Geometry: see drawing. Coordinates: mm, zero at the bounding-box minimum. Give positions to 0.01 mm unless a question says otherwise; leave off trailing zeros. Write each loop counter-clockwise with the first axis right and the second up, starting at its lowest first coordinate (ties: lowest second). Pieces come first, ordered by that corner, then holes. Notation, with made-up numbers: M 52,66.25 L 95,66.25 A13 ccw 95,76.25 Z; hole C 49,86.5 d1. An arc over 180 degrees is marked long. Use CSV: the item, a comma, the result in double quotes. Start each with the question number.
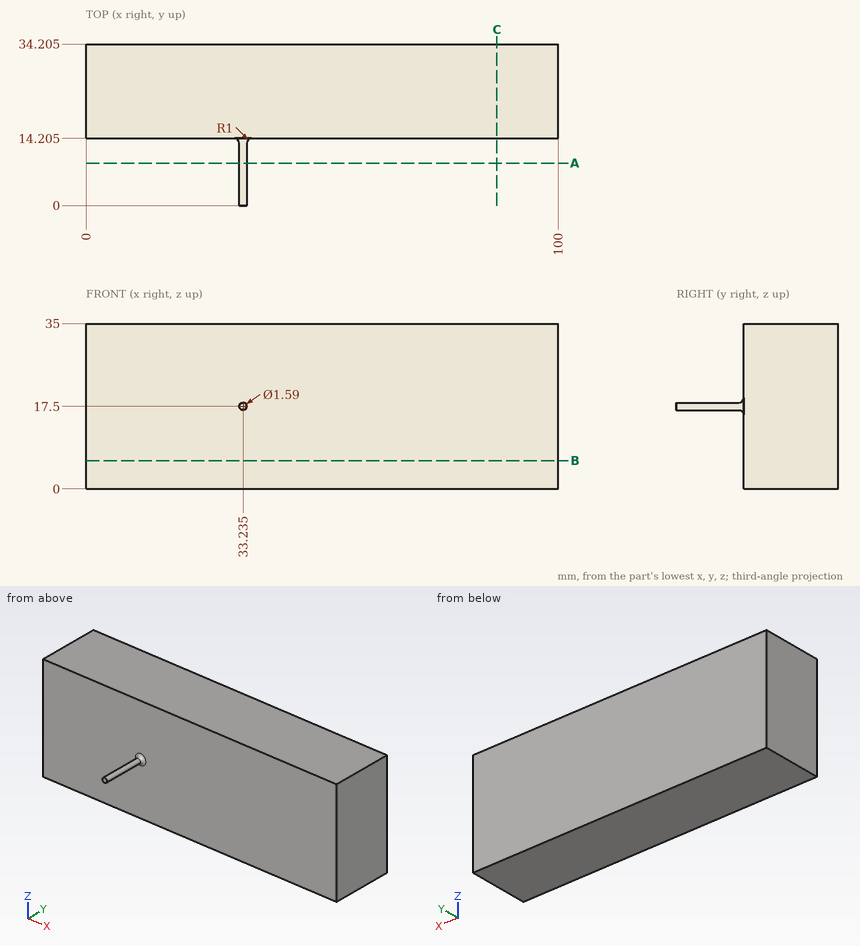
1. Section B-B on z = 6. Return loops of the section in (x, y) (3 decimals).
2. Section A-A on y = 9. Return loops of the section in (x, z) (3 decimals).
3. Section C-C on x = 87. Return loops of the section in (y, z) (3 decimals), then the cut area to 3 significant figures.
4. Line query: probe 1 along Y at (x, z) = (12, 31.5) (3 decimals). Output: solid intervals per line, ascending.
5. First-contact query: pin 1 (3 mm diameter, centred on x = 62.5, z = 23.5, fed in from -Y) (3 decimals). Flat tip, straight axial feed; report the tip coordinate or a pass-through.
Resolved:
1,outline,"M 0,14.205 L 100,14.205 L 100,34.205 L 0,34.205 Z"
2,outline,"C 33.235,17.5 d1.59"
3,outline,"M 14.205,0 L 34.205,0 L 34.205,35 L 14.205,35 Z"
3,area,"700 mm2"
4,probe 1,"y = 14.205 to 34.205"
5,pin 1,"stops at y = 14.205"
